Can you work these out from the model? Positions are in its coordinate system, mm. A direction names the side the tool comes from. Round coordinates to 2 decimals unless told otherwise and drop trailing zeros. Order: outer loops, then holes, each group sorted by start corner. A loop starts at its lowest first (then second) coordinate and runs counter-clockwise, first axis right, second up. Notation, with made-up numbers: (83.25, 2.5) - (131.25, 2.5) arc R29 ccw to (131.25, 33.5) - close; hole circle Ø7 at (61.25, 10.25). An arc over 180 degrees is marked (long way). Write item = value, one per line.
from build123d import *

# Parameters (mm, degrees)
F0_W            = 12
F0_H            = 2
F1_DEPTH        = 3
F2_W            = 3
F2_H            = 29
F3_DEPTH        = 29
F4_W            = 15
F4_H            = 2
F5_DEPTH        = 15
F6_SIZE         = 14.99999
F8_D            = 3.5
F10_D           = 3.5
F10_CSINK_D     = 7
F10_CSINK_ANGLE = 90
F11_R           = 7.5
F11_R_2         = 5
F12_DEPTH       = 25
F13_W           = 10
F13_H           = 12
F14_DEPTH       = 68.001


# Not quite as in the source:
# - a fillet or chamfer is up to 0.001 mm smaller than in the source, because OpenCascade refuses the exact size
# - a feature names something its author has since deleted; it is built from what else it names


with BuildPart() as f1:
    # F0 (on Top) → F1 (new body)
    with BuildSketch(Plane.XY):
        Polygon((34, -12.5), (34, 16.5), (8, 16.5), (-8, 16.5), (-34, 16.5), (-34, -12.5), (-21, -12.5), (-9, -12.5), (9, -12.5), (21, -12.5), align=None)
        with BuildLine():
            Line((-8, 16.5), (8, 16.5))
            ThreePointArc((8, 16.5), (0, 24.5), (-8, 16.5))
        make_face()
        with Locations((-15, -13.5)):
            Rectangle(F0_W, F0_H)
        with Locations((15, -13.5)):
            Rectangle(F0_W, F0_H)
    extrude(amount=F1_DEPTH)

    # F2 (on face) → F3 (join)
    with BuildSketch(Plane.XY.offset(3)):
        with Locations((-32.5, 2)):
            Rectangle(F2_W, F2_H)
        with Locations((32.5, 2)):
            Rectangle(F2_W, F2_H)
    extrude(amount=F3_DEPTH)

    # F4 (on face) → F5 (join)
    with BuildSketch(Plane.XY.offset(3)):
        with Locations((-23.5, 15.5)):
            Rectangle(F4_W, F4_H)
        with Locations((23.5, 15.5)):
            Rectangle(F4_W, F4_H)
    extrude(amount=F5_DEPTH)

    # F6 (size 15 in the source; OpenCascade refuses exactly that, so slightly less here)
    f6_edges = [f1.edges().sort_by_distance(p)[0] for p in [
        (-16, 15.5, 18),
        (16, 15.5, 18),
    ]]
    chamfer(f6_edges, length=F6_SIZE)

    # F8 (through all)
    with Locations(Plane(origin=(-34, 0, 0), x_dir=(0, -1, 0), z_dir=(-1, 0, 0))):
        with Locations((10, 29.5), (10, 9.5), (-10, 9.5), (-10, 29.5)):
            Hole(F8_D / 2)

    # F10 (through all)
    with Locations(Plane.XY.offset(3)):
        with Locations((0, 18), (-15.5884572681, -9), (15.5884572681, -9)):
            CounterSinkHole(F10_D / 2, F10_CSINK_D / 2, counter_sink_angle=F10_CSINK_ANGLE)

    # F11 (on face) → F12 (cut)
    with BuildSketch(Plane(origin=(0, 0, 0), x_dir=(1, 0, 0), z_dir=(0, 0, -1))):
        Circle(F11_R)
        with Locations((20, 0)):
            Circle(F11_R_2)
        with Locations((-20, 0)):
            Circle(F11_R_2)
    extrude(amount=-F12_DEPTH, mode=Mode.SUBTRACT)

    # F13 (on face) → F14 (cut, through all)
    with BuildSketch(Plane.YZ.offset(34)):
        with Locations((0, 26)):
            Rectangle(F13_W, F13_H)
        with BuildLine():
            ThreePointArc((-5, 20), (0, 15), (5, 20))
            Line((5, 20), (-5, 20))
        make_face()
    extrude(amount=-F14_DEPTH, mode=Mode.SUBTRACT)


solid = f1.part
(1) Will these pins go through, and if not, where does the flat tip stop? P1, Ø2.5, axis at x = 33, z = 28, coming from the +Y side; P2, Ø8.5, axis at y = 0.5, z = 20, coming from the -X side (3 decimals); P3, Ø2, axis at y = -14, z = 1.5, coming from the -X side; P4, Ø14.5, axis at x = 28.5, z = 9.5, coming from the -Y side.
Computed:
P1 = 16.5
P2 = through
P3 = -21
P4 = -12.5
(2) Thinking about a two-plate mould opening in Z: for faces 4 (the face through (-27, 16.5, 9)), 5 (the face through (-32.5, -9.1, 11)), 6 (the face through (33, 0, 15)), which applies, +Z half, -Z half, draft (parallel to the pull), parting line (faces both ways), or undercut?
Computed:
face_4 = draft
face_5 = undercut
face_6 = +Z half
(3) On a 3-axis mill with a long thin cutter (end or side, diameter ignored), from which of +Z, -Z, +X, -X, +Y, -Y can I reach the whole of each face in a straight line? I mean faces 1 (the face through (-25, 14.5, 9)), 2 (the face through (0, -12.5, 1)), 3 (the face through (-32, 5, 26)). Say none if no direction works.
Computed:
face_1 = +Z, -Y
face_2 = +Z, -Z, -Y
face_3 = +Z, +X, -X
(4) If I drill on line 1 (Z direction, x = -32.8, y = -10); line 2 (Y direction, x = 0, z = 1); line 3 (X direction, y = -4.5, z = 16.5), over which ranges is the centre line in solid material (lowest first)? Write a range as from..to.
Computed:
line_1 = 0..7.75, 11.25..27.75, 31.25..32
line_2 = -12.5..-7.5, 7.5..16.25, 19.75..24.5
line_3 = -34..-31, 31..34
(5) If we section it at C-C (x = 0): Write out the boundary of the cut face in (y, z), plus the area to 3 significant figures.
Computed:
outline = (-12.5, 0) - (-7.5, 0) - (-7.5, 3) - (-12.5, 3) - close; (7.5, 0) - (16.25, 0) - (16.25, 1.25) - (14.5, 3) - (7.5, 3) - close; (19.75, 0) - (24.5, 0) - (24.5, 3) - (21.5, 3) - (19.75, 1.25) - close
area = 52.4 mm^2
(6) If we section it at D-D (z = 29.5): State how many separate pieces and enclosed holes the cut face has, plus the area to 3 significant figures.
Computed:
separate_pieces = 8
enclosed_holes = 0
area = 72.0 mm^2
(7) If we section it at A-A (z = 23): Write out the boundary of the cut face in (x, y), plus the area to 3 significant figures.
Computed:
outline = (-34, -12.5) - (-31, -12.5) - (-31, -5) - (-34, -5) - close; (-34, 5) - (-31, 5) - (-31, 16.5) - (-34, 16.5) - close; (31, -12.5) - (34, -12.5) - (34, -5) - (31, -5) - close; (31, 5) - (34, 5) - (34, 16.5) - (31, 16.5) - close
area = 114 mm^2
(8) If we section it at B-B (y = 10): Write out the boundary of the cut face in (x, z).
Computed:
outline = (-34, 0) - (34, 0) - (34, 7.75) - (31, 7.75) - (31, 3) - (-31, 3) - (-31, 7.75) - (-34, 7.75) - close; (-34, 11.25) - (-31, 11.25) - (-31, 27.75) - (-34, 27.75) - close; (-34, 31.25) - (-31, 31.25) - (-31, 32) - (-34, 32) - close; (31, 11.25) - (34, 11.25) - (34, 27.75) - (31, 27.75) - close; (31, 31.25) - (34, 31.25) - (34, 32) - (31, 32) - close
